```python
from build123d import *

# Parameters (mm, degrees)
ESQUISSE1_R        = 8.15
ESQUISSE1_R_2      = 2
BOSS_EXTRU_1_DEPTH = 5


with BuildPart() as part:
    # Esquisse1 → Boss.-Extru.1 (new body)
    # profile 1 of 7: a face of its own
    with BuildSketch(Plane.XY):
        Polygon((-30, 20), (-30, -20), (30, -20), (30, 20), (15, 20), (15, 15), (-15, 15), (-15, 20), align=None)
        with Locations((-12.7, 0)):
            Circle(ESQUISSE1_R, mode=Mode.SUBTRACT)
        with Locations((12.7, 0)):
            Circle(ESQUISSE1_R, mode=Mode.SUBTRACT)
    # profile 2 of 7: a face of its own
    with BuildSketch(Plane.XY):
        with BuildLine():
            Line((-3.122498999, 20), (-15, 20))
            Line((-15, 20), (-15, 15))
            Line((-15, 15), (15, 15))
            Line((15, 15), (15, 20))
            Line((15, 20), (3.122498999, 20))
            ThreePointArc((3.122498999, 20), (0, 18.5), (-3.122498999, 20))
        make_face()
    # profile 3 of 7: a face of its own
    with BuildSketch(Plane.XY):
        with BuildLine():
            Line((-15, 25), (-15, 20))
            Line((-15, 20), (-3.122498999, 20))
            ThreePointArc((-3.122498999, 20), (-4, 22.5), (-3.122498999, 25))
            Line((-3.122498999, 25), (-15, 25))
        make_face()
    # profile 4 of 7: a face of its own
    with BuildSketch(Plane.XY):
        with BuildLine():
            Line((3.122498999, 20), (15, 20))
            Line((15, 20), (15, 25))
            Line((15, 25), (3.122498999, 25))
            ThreePointArc((3.122498999, 25), (3.774254628, 23.824764885), (4, 22.5))
            ThreePointArc((4, 22.5), (3.774254628, 21.175235115), (3.122498999, 20))
        make_face()
    # profile 5 of 7: a face of its own
    with BuildSketch(Plane.XY):
        with BuildLine():
            Line((3.122498999, 20), (-3.122498999, 20))
            ThreePointArc((-3.122498999, 20), (0, 18.5), (3.122498999, 20))
        make_face()
    # profile 6 of 7: a face of its own
    with BuildSketch(Plane.XY):
        with BuildLine():
            ThreePointArc((-3.122498999, 25), (-4, 22.5), (-3.122498999, 20))
            Line((-3.122498999, 20), (3.122498999, 20))
            ThreePointArc((3.122498999, 20), (3.774254628, 21.175235115), (4, 22.5))
            ThreePointArc((4, 22.5), (3.774254628, 23.824764885), (3.122498999, 25))
            Line((3.122498999, 25), (-3.122498999, 25))
        make_face()
        with Locations((0, 22.5)):
            Circle(ESQUISSE1_R_2, mode=Mode.SUBTRACT)
    # profile 7 of 7: a face of its own
    with BuildSketch(Plane.XY):
        with BuildLine():
            ThreePointArc((3.122498999, 25), (0, 26.5), (-3.122498999, 25))
            Line((-3.122498999, 25), (3.122498999, 25))
        make_face()
    extrude(amount=BOSS_EXTRU_1_DEPTH)


solid = part.part
```
Design review of the part built by this model. Coordinates are the model's own, in mm. A direction names the side the tool comes from. Give positions to 0.01 mm unless a question says otherwise; leave off trailing zeros. Write each loop counter-clockwise with the first axis right and the second up, starting at its lowest first coordinate (ties: lowest second). Pieces come first, ordered by that corner, then holes. Notation, with made-up numbers: (-14.5, 83.25) -> (29.5, 83.25) arc R23 ccw to (29.5, 110.25) -> close; hole circle Ø9 at (73, -17). An arc over 180 degrees is marked (long way). Answer in a Markdown table with one row per item.
(1) To check wall thickness, follow probe 1 along Y at (x, z) = (0, 1.4); probe 2 along Y at (x, z) = (-12.7, 2.4); probe 3 along Y at (x, z) = (21, 0.9). State the ranges of each line that lie inside material, in increasing order.
Results:
| item | result |
|---|---|
| probe 1 | -20 to 20.5, 24.5 to 26.5 |
| probe 2 | -20 to -8.15, 8.15 to 25 |
| probe 3 | -20 to 20 |
(2) Consider section A-A (x = 12.7). State the section outline as (y, z) points.
Results:
| item | result |
|---|---|
| outline | (-20, 0) -> (-8.15, 0) -> (-8.15, 5) -> (-20, 5) -> close; (8.15, 0) -> (25, 0) -> (25, 5) -> (8.15, 5) -> close |
(3) Clearance check with a flat-ended pin moving along its axis: pin 1 (2.5 mm diameter, centred on x = -20.5, z = 1.5, fed in from +Y). State where the tip first meets the part, or that it passes through.
Results:
| item | result |
|---|---|
| pin 1 | y = 20 |
(4) Consider section B-B (z = 2.6). State the section outline as (x, y) points.
Results:
| item | result |
|---|---|
| outline | (-30, -20) -> (30, -20) -> (30, 20) -> (15, 20) -> (15, 25) -> (3.12, 25) arc R4 ccw to (-3.12, 25) -> (-15, 25) -> (-15, 20) -> (-30, 20) -> close; hole circle Ø16.3 at (-12.7, 0); hole circle Ø4 at (0, 22.5); hole circle Ø16.3 at (12.7, 0) |
(5) For faces 5 (the flat face through (9, 25, 2)), 6 (the flat face through (-22, 20, 2)), 7 (the flat face through (-30, 0, 2)), list the 3-axis set-ups (+Z, -Z, +X, -X, +Y, -Y) from which the entire face can be reached by the end or side of a thin tool; tool diameter is ignored.
Results:
| item | result |
|---|---|
| face 5 | +Z, -Z, +X, +Y |
| face 6 | +Z, -Z, -X, +Y |
| face 7 | +Z, -Z, -X, +Y, -Y |
(6) Mouldability with a two-part tool opening along Y and no side actions: class faces 1 (the flat face through (-9, 25, 2)), 2 (the cylindrical face through (-20.842, 0.358, 2.465)), 3 (the flat face through (15, 22, 2)), 4 (the flat face through (0, -20, 2)) as +Y half, -Y half, draft (parallel to the pull), parting line (faces both ways), or undercut.
Results:
| item | result |
|---|---|
| face 1 | +Y half |
| face 2 | undercut |
| face 3 | draft |
| face 4 | -Y half |
(7) Consider section C-C (y = 22.5). State the section outline as (x, z) points.
Results:
| item | result |
|---|---|
| outline | (-15, 0) -> (-2, 0) -> (-2, 5) -> (-15, 5) -> close; (2, 0) -> (15, 0) -> (15, 5) -> (2, 5) -> close |
(8) Consider section D-D (y = -3.5). State the section outline as (x, z) points, then the cut area to 3 significant figures.
Results:
| item | result |
|---|---|
| outline | (-30, 0) -> (-20.06, 0) -> (-20.06, 5) -> (-30, 5) -> close; (-5.34, 0) -> (5.34, 0) -> (5.34, 5) -> (-5.34, 5) -> close; (20.06, 0) -> (30, 0) -> (30, 5) -> (20.06, 5) -> close |
| area | 153 mm2 |
